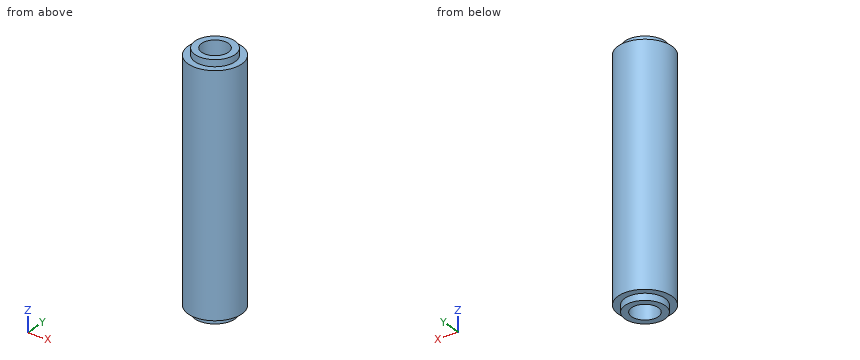
Autodesk Inventor part; units mm, degrees
ref_plane "YZ Plane" through (0, 0, 0) normal (1, 0, 0) x (0, 1, 0)
ref_plane "XZ Plane" through (0, 0, 0) normal (0, 1, 0) x (-1, 0, 0)
ref_plane "XY Plane" through (0, 0, 0) normal (0, 0, 1) x (1, 0, 0)
sketch "Sketch1" plane through (0, 0, 0) normal (0, 0, 1) x (1, 0, 0)
  circle A0 centre (0, 0) radius 6.35
  circle A1 centre (0, 0) radius 3.175
  dimension "d0" = 12.7
  dimension "d13" = 3.175
extrude "Base" add sketch "Sketch1" along normal mid plane 58.7375
sketch "Sketch4" plane through (0, 0, 29.3688) normal (0, 0, 1) x (1, 0, 0)
  circle A0 centre (0, 0) radius 6.35
  circle A1 centre (0, 0) radius 4.7625
  dimension "d16" = 9.525
extrude "Extrusion4" cut sketch "Sketch4" against normal blind 1.5875
mirror "Mirror2" about plane through (0, 0, 0) normal (0, 0, 1) of "Extrusion4"
properties part number "gearbox_standoff" material "Aluminum-6061"
Geometry: final body of the model. Coordinates: model frame, mm. Round coordinates to 2 decimals unless told otherwise and drop trailing zeros. Write each loop counter-clockwise with the first axis right and the second up, starting at its lowest first coordinate (ties: lowest second). Pieces come first, ordered by that corner, then holes.
Item 1: Pin query (flat end, axial travel): P1, Ø7.5, axis at x = 0, y = 0, coming from the +Z side; P2, Ø1.5, axis at y = 1.5, z = -7, coming from the -X side; P3, Ø1, axis at y = -4.5, z = -16, coming from the +X side. Return the tip coordinate at first contact, or that it passes through.
Item 2: Material intervals for L1, parallel to Y at x = 0, z = 8 (3 decimals); L2, parallel to Z at x = 4.5, y = -2; L3, parallel to Y at x = 0.5, z = -14, sorted ascending.
Item 3: Section query D-D (z = 9). Return loops of the section in (x, y) (3 decimals).
Item 4: Section query C-C (x = -3.75). Return loops of the section in (y, z), plus the area to 3 significant figures.
Completed:
1. P1: stops at z = 29.37
1. P2: stops at x = -6.31
1. P3: stops at x = 4.93
2. L1: y = -6.35 to -3.175, 3.175 to 6.35
2. L2: z = -27.78 to 27.78
2. L3: y = -6.33 to -3.14, 3.14 to 6.33
3. outline: circle Ø12.7 at (0, 0); hole circle Ø6.35 at (0, 0)
4. outline: (-5.12, -27.78) - (-2.94, -27.78) - (-2.94, -29.37) - (2.94, -29.37) - (2.94, -27.78) - (5.12, -27.78) - (5.12, 27.78) - (2.94, 27.78) - (2.94, 29.37) - (-2.94, 29.37) - (-2.94, 27.78) - (-5.12, 27.78) - close
4. area: 588 mm2
